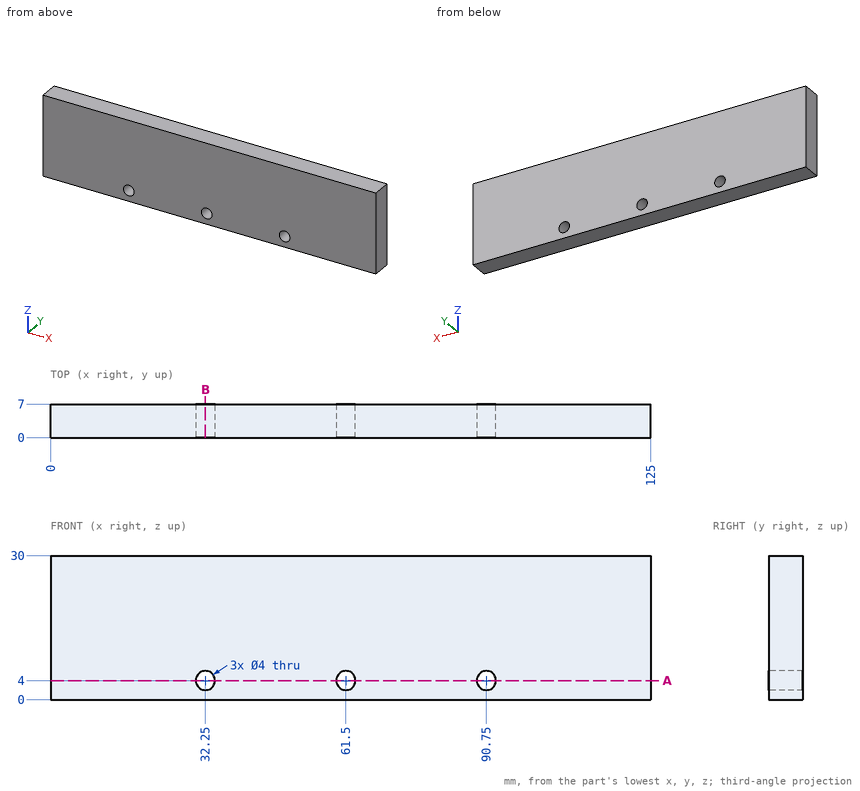
Part print with two shaded views. Sizes in mm from the minimum x, y, z corner. Round coordinates to 2 decimals unless told otherwise and drop trailing zeros. Write each loop counter-clockwise with the first axis right and the second up, starting at its lowest first coordinate (ties: lowest second). Pieces come first, ordered by that corner, then holes. Notation, with made-up numbers: (14, -1.5) -> (63, -1.5) arc R24 cw to (63, 12.5) -> close; hole circle Ø10 at (39, -26). An arc over 180 degrees is marked (long way). Use one line per item in the form item = value.
Q1. Drill centre lines: L1, parallel to Z at x = 32.25, y = 4.5; L2, parallel to X at y = 2.5, z = 3.5. Where is each one in solid material? Low to high.
Conclusion:
L1 = 0 to 2, 6 to 30
L2 = 0 to 30.31, 34.19 to 59.56, 63.44 to 88.81, 92.69 to 125
Q2. Band-saw the part on B-B, the plane x = 32.25. Write the cut outline in (y, z).
Conclusion:
outline = (0, 0) -> (7, 0) -> (7, 2) -> (0, 2) -> close; (0, 6) -> (7, 6) -> (7, 30) -> (0, 30) -> close
Q3. Band-saw the part on A-A, the plane z = 4. Write the cut outline in (x, y), then the cut area to 3 significant figures.
Conclusion:
outline = (0, 0) -> (30.25, 0) -> (30.25, 7) -> (0, 7) -> close; (34.25, 0) -> (59.5, 0) -> (59.5, 7) -> (34.25, 7) -> close; (63.5, 0) -> (88.75, 0) -> (88.75, 7) -> (63.5, 7) -> close; (92.75, 0) -> (125, 0) -> (125, 7) -> (92.75, 7) -> close
area = 791 mm²
Q4. Drop a flat-ended pin along its axis: P1, Ø4, axis at x = 36, z = 18.5, coming from the -Y side. Give the stop position or say it passes through.
Conclusion:
P1 = 0
